Could you check a few things on this model? Use its own coordinates, in mm. A direction names the side the tool comes from. Round coordinates to 2 decimals unless told otherwise and drop trailing zeros. Order: outer loops, then holes, each group sorted by start corner. A loop starts at its lowest first (then second) coordinate and runs counter-clockwise, first axis right, second up.
```python
from build123d import *

# Parameters (mm, degrees)
F2_SIZE         = 1
F3_R            = 4
F4_DEPTH        = 15
F4_COPIES_COUNT = 3
F6_D            = 4
F6_DEPTH        = 12
F6_TIP          = 1.2017212381


# Not quite as in the source:
# - a pattern or mirror of a feature is missing from the dataset's text; its kind, count and spacing are read off the source's solid


with BuildPart() as f1:
    # F0 (on Right) → F1 (revolve)
    with BuildSketch(Plane.YZ):
        with BuildLine():
            Line((0, 11), (0, 5))
            Line((0, 5), (25, 5))
            Line((25, 5), (25, 36))
            Line((25, 36), (5, 36))
            Line((5, 36), (5, 31))
            Line((5, 31), (7, 31))
            ThreePointArc((7, 31), (9.1213203436, 30.1213203436), (10, 28))
            Line((10, 28), (10, 14))
            ThreePointArc((10, 14), (9.1213203436, 11.8786796564), (7, 11))
            Line((7, 11), (0, 11))
        make_face()
    revolve(axis=Axis((0, 9.0291841974, 0), (0, 1, 0)))

    # F2
    f2_edges = [f1.edges().sort_by_distance(p)[0] for p in [
        (0, 0, -5),
    ]]
    chamfer(f2_edges, length=F2_SIZE)

    # F3 (on face) → F4 (cut, through all)
    with BuildSketch(Plane(origin=(0, 25, 0), x_dir=(-1, 0, 0), z_dir=(0, 1, 0))):
        with Locations((0, 21)):
            Circle(F3_R)
    f4 = extrude(amount=-F4_DEPTH, mode=Mode.SUBTRACT)

    # F4_copies: F4 ×3 about axis
    f4_copies_axis = Axis((0, 0, 0), (0, 1, 0))
    for i in range(1, F4_COPIES_COUNT):
        add(f4.rotate(f4_copies_axis, i * 360 / F4_COPIES_COUNT), mode=Mode.SUBTRACT)

    # F6
    with Locations(Plane(origin=(0, 25, 0), x_dir=(-1, 0, 0), z_dir=(0, 1, 0))):
        with Locations((0, 5)):
            Hole(F6_D / 2, depth=F6_DEPTH)
            with Locations((0, 0, -(F6_DEPTH + F6_TIP / 2))):  # 118° drill point
                Cone(0, F6_D / 2, F6_TIP, mode=Mode.SUBTRACT)


solid = f1.part
```
Q1. I need wall thicknesses on L1, parallel to X at y = 5.75, z = -1; L2, parallel to Z at x = 6, y = 5.5; L3, parallel to X at y = 18.75, z = 0. Which ranges of each line are inside material? Lowest first, please.
Q2. We'd pull the mould along X, two halves only. Please class faces 3 (the cylindrical face through (0, 19, 7)), 4 (the flat face through (-5, 0, 5)), 5 (the cylindrical face through (35.694, 14.86, -4.686)): released by +X, released by -X, zero draft, split by the parting line, or undercut.
Q3. Imagine slicing it at D-D, the plane y = 18.5. Please give me the cut outline in (x, z), then the cut area to 3 significant figures.
Q4. For P1, Ø1.5, axis at y = 12.5, z = -4.5, coming from the +X side; P2, Ø4, axis at y = 14.5, z = 24.5, coming from the -X side; P3, Ø6.5, axis at x = 0, z = 21, coming from the -Y side; P4, Ø6.5, axis at x = 0, z = 5, coming from the -Y side, each with a flat end and sliding along its axis, tell me the tip position at first contact or that it passes through.
Q5. Imagine slicing it at A-A, the plane x = 0. Please give me the cut outline in (y, z).
Q6. Imagine slicing it at B-B, the plane z = 0. Please give me the cut outline in (x, y).
Q7. For faces 1 (the conical face through (-0.02, 12.274, 5.792)), 2 (the cylindrical face through (-10.74, 3.45, -2.38)), which set-ups out of +Z, -Z, +X, -X, +Y, -Y let a thin tool reach every point of the face, with its end or its side?
Q8. Imagine slicing it at C-C, the plane y = 2. Please give me the cut outline in (x, z).
Filled in:
1. L1: x = -35.99 to -30.98, -10.95 to -4.9, 4.9 to 10.95, 30.98 to 35.99
1. L2: z = -35.5 to -30.41, -9.22 to 9.22, 30.41 to 35.5
1. L3: x = -36 to -5, 5 to 36
2. face 3: undercut
2. face 4: zero draft
2. face 5: split by the parting line
3. outline: circle Ø72 at (0, 0); hole circle Ø8 at (-18.19, -10.5); hole circle Ø8 at (0, 21); hole (-1.96, 4.6) arc R5 ccw (long way) to (1.96, 4.6) arc R2 ccw (long way) to start; hole circle Ø8 at (18.19, -10.5)
3. area: 3,840 mm2
4. P1: stops at x = 35.8
4. P2: stops at x = -28.1
4. P3: passes through
4. P4: stops at y = 0
5. outline: (0, -11) - (7, -11) arc R3 cw to (10, -14) - (10, -28) arc R3 cw to (7, -31) - (5, -31) - (5, -36) - (25, -36) - (25, -5) - (1, -5) - (0, -6) - close; (0, 6) - (1, 5) - (11.8, 5) - (13, 7) - (25, 7) - (25, 17) - (10, 17) - (10, 14) arc R3 cw to (7, 11) - (0, 11) - close; (5, 31) - (7, 31) arc R3 cw to (10, 28) - (10, 25) - (25, 25) - (25, 36) - (5, 36) - close
6. outline: (-36, 5) - (-31, 5) - (-31, 7) arc R3 cw to (-28, 10) - (-14, 10) arc R3 cw to (-11, 7) - (-11, 0) - (-6, 0) - (-5, 1) - (-5, 25) - (-36, 25) - close; (5, 1) - (6, 0) - (11, 0) - (11, 7) arc R3 cw to (14, 10) - (28, 10) arc R3 cw to (31, 7) - (31, 5) - (36, 5) - (36, 25) - (5, 25) - close
7. face 1: +Y
7. face 2: -Y
8. outline: circle Ø22 at (0, 0); hole circle Ø10 at (0, 0)
